```python
from build123d import *

# Parameters (mm, degrees)
BOSS_EXTRUDE1_DEPTH             = 14.2875
SKETCH2_R                       = 5.9436
BOSS_EXTRUDE2_DEPTH             = 0.889
SKETCH3_R                       = 6.35
BOSS_EXTRUDE3_DEPTH             = 2.54
CHAMFER1_SIZE                   = 0.762
BOSS_EXTRUDE4_DEPTH             = 43.0149
BOSS_EXTRUDE5_START             = 0.889
SKETCH6_R                       = 5.9436
BOSS_EXTRUDE5_DEPTH             = 0.889
BOSS_EXTRUDE6_START             = 2.54
SKETCH7_R                       = 6.35
BOSS_EXTRUDE6_DEPTH             = 2.54
CHAMFER2_SIZE                   = 0.762
F_1_4_0_25_DIAMETER_HOLE1_D     = 6.35
F_1_4_0_25_DIAMETER_HOLE1_DEPTH = 6.35
F_1_4_0_25_DIAMETER_HOLE1_TIP   = 1.907732465


with BuildPart() as part:
    # Sketch1 → Boss-Extrude1 (new, symmetric)
    with BuildSketch(Plane.XY):
        Polygon((7.332348419, 0), (3.666174209, 6.35), (-3.666174209, 6.35), (-7.332348419, 0), (-3.666174209, -6.35), (3.666174209, -6.35), align=None)
    extrude(amount=BOSS_EXTRUDE1_DEPTH, both=True)

    # Sketch2 → Boss-Extrude2 (add)
    with BuildSketch(Plane(origin=(0, 0, -14.2875), x_dir=(-1, 0, 0), z_dir=(0, 0, -1))):
        with Locations(Location((0, 0, 0), (0, 0, 180))):
            Circle(SKETCH2_R)
    extrude(amount=BOSS_EXTRUDE2_DEPTH)

    # Sketch3 → Boss-Extrude3 (add)
    with BuildSketch(Plane(origin=(0, 0, -15.1765), x_dir=(-1, 0, 0), z_dir=(0, 0, -1))):
        Circle(SKETCH3_R)
    extrude(amount=BOSS_EXTRUDE3_DEPTH)

    # Chamfer1
    chamfer1_edges = [part.edges().sort_by_distance(p)[0] for p in [
        (6.35, 0, -17.7165),
    ]]
    chamfer(chamfer1_edges, length=CHAMFER1_SIZE)

    # Sketch5 → Boss-Extrude4 (add)
    with BuildSketch(Plane.XY.offset(14.2875)):
        Polygon((3.666174209, 6.35), (-3.666174209, 6.35), (-7.332348419, 0), (-3.666174209, -6.35), (3.666174209, -6.35), (7.332348419, 0), align=None)
    extrude(amount=BOSS_EXTRUDE4_DEPTH)

    # Sketch6 → Boss-Extrude5 (add)
    with BuildSketch(Plane.XY.offset(57.3024).offset(BOSS_EXTRUDE5_START)):
        Circle(SKETCH6_R)
    extrude(amount=-BOSS_EXTRUDE5_DEPTH)

    # Sketch7 → Boss-Extrude6 (add)
    with BuildSketch(Plane.XY.offset(58.1914).offset(BOSS_EXTRUDE6_START)):
        with Locations(Location((0, 0, 0), (0, 0, 180))):
            Circle(SKETCH7_R)
    extrude(amount=-BOSS_EXTRUDE6_DEPTH)

    # Chamfer2
    chamfer2_edges = [part.edges().sort_by_distance(p)[0] for p in [
        (6.35, 0, 60.7314),
    ]]
    chamfer(chamfer2_edges, length=CHAMFER2_SIZE)

    # 1/4 (0.25) Diameter Hole1
    with Locations(Plane.XY.offset(60.7314)):
        with Locations((0, 0)):
            Hole(F_1_4_0_25_DIAMETER_HOLE1_D / 2, depth=F_1_4_0_25_DIAMETER_HOLE1_DEPTH)
            with Locations((0, 0, -(F_1_4_0_25_DIAMETER_HOLE1_DEPTH + F_1_4_0_25_DIAMETER_HOLE1_TIP / 2))):  # 118° drill point
                Cone(0, F_1_4_0_25_DIAMETER_HOLE1_D / 2, F_1_4_0_25_DIAMETER_HOLE1_TIP, mode=Mode.SUBTRACT)


solid = part.part
```
Input: part model. Units: mm. Frame: model coordinates. A direction names the side the tool comes from. Round coordinates to 2 decimals unless told otherwise and drop trailing zeros. Order: outer loops, then holes, each group sorted by start corner. A loop starts at its lowest first (then second) coordinate and runs counter-clockwise, first axis right, second up. Notation, with made-up numbers: (-22.75, 47) - (10.25, 47) arc R27 cw to (10.25, 65) - close; hole circle Ø9 at (14.25, 35). An arc over 180 degrees is marked (long way). Answer in a Markdown table with one row per item.
Item 1: Line query: line 1 (Y direction, x = 0, z = 55.5) (3 decimals); line 2 (X direction, y = 0, z = 57.25) (3 decimals). Output: solid intervals per line, ascending.
Model answer:
| item | result |
|---|---|
| line 1 | y = -6.35 to -3.175, 3.175 to 6.35 |
| line 2 | x = -7.332 to -3.175, 3.175 to 7.332 |
Item 2: Mould query, pull axis X, two halves, no side actions, for faces 6 (the cylindrical face through (5.669, -1.785, -14.726)), 7 (the conical face through (-0.12, -0.538, 52.805)), 8 (the flat face through (5.525, 3.131, 21.006)). Classes: released by +X, released by -X, zero draft, split by the parting line, or undercut.
Model answer:
| item | result |
|---|---|
| face 6 | split by the parting line |
| face 7 | undercut |
| face 8 | released by +X |
Item 3: Section query A-A (z = 51). Return the cut outline in (x, y).
Model answer:
| item | result |
|---|---|
| outline | (-7.33, 0) - (-3.67, -6.35) - (3.67, -6.35) - (7.33, 0) - (3.67, 6.35) - (-3.67, 6.35) - close |
Item 4: Reachability of faces 1 (the cylindrical face through (-2.93, 5.634, 59.093)), 2 (the flat face through (0, -6.35, 21)), 3 (the cylindrical face through (5.669, 1.785, 57.753)), 4 (the cylindrical face through (1.38, -6.2, -16.05)), 5 (the flat face through (-5.525, -3.131, 21.006)) from +Z, -Z, +X, -X, +Y, -Y: full face, straight path, thin tool, end or side. Return the list, or none.
Model answer:
| item | result |
|---|---|
| face 1 | +Z |
| face 2 | +Z, -Z, +X, -X, -Y |
| face 3 | none |
| face 4 | -Z |
| face 5 | +Z, -Z, -X, -Y |
Item 5: Pin query (flat end, axial travel): pin 1 (1 mm diameter, centred on y = 3, z = 2, fed in from +X); pin 2 (4 mm diameter, centred on y = -4.5, z = -7.5, fed in from -X); pin 3 (4 mm diameter, centred on x = 0, y = 0, fed in from +Z). Return the tip coordinate at first contact, or that it passes through.
Model answer:
| item | result |
|---|---|
| pin 1 | stops at x = 5.89 |
| pin 2 | stops at x = -5.89 |
| pin 3 | stops at z = 53.68 |
